Here's how the part is built. I have some questions about the finished solid (model axes, mm). Coordinates: 2 decimals unless noted, no trailing zeros. Write each loop counter-clockwise with the first axis right and the second up, starting at its lowest first coordinate (ties: lowest second). Pieces come first, ordered by that corner, then holes. Notation, with made-up numbers: (44, 50.5) -> (61, 50.5) arc R27 ccw to (61, 81.5) -> close; hole circle Ø11 at (48, 0.25). An arc over 180 degrees is marked (long way). Use a Markdown table: item, result. Add a question column.
Item 1: Imagine slicing it at B-B, the plane y = 0. Write out the boundary of the cut face in (x, z).
Item 2: Will this pin go through, and if not, where does the flat tip stop? pin 1 Ø6.5 at (y, z) = (0, 12.7) entering from -X.
Item 3: Imagine slicing it at A-A, the plane z = 352.7. Write out the boundary of the cut face in (x, y), and give its area (3 significant figures).
Item 4: If I drill on line 1 along Y through (x, z) = (0.75, 352.7); line 2 along Z through (x, y) = (-11.25, 1.5); line 3 along Z through (x, y) = (-1.25, 2.25), over which ranges is the centre line in solid material (lowest first)? Write a range as from..to.
Item 5: If we mould it in two halves opening along Y, with no side actions, what happens to faces 1 (the flat face through (0, 12.7, 180)), 2 (the flat face through (0, 0, 365.4)), 3 (the cylindrical face through (-0.18, 1.05, 356.04))? For each: pulls with the +Y half, pulls with the -Y half, needs draft (parallel to the pull), parting line crosses it, or undercut.
```python
from build123d import *

# Parameters (mm, degrees)
SKETCH1_W           = 25.4
SKETCH1_H           = 25.4
BOSS_EXTRUDE1_DEPTH = 365.4
SKETCH10_R          = 3.5
CUT_EXTRUDE6_DEPTH  = 367.501855384


with BuildPart() as part:
    # Sketch1 → Boss-Extrude1 (new body)
    with BuildSketch(Plane.XY):
        Rectangle(SKETCH1_W, SKETCH1_H)
    extrude(amount=BOSS_EXTRUDE1_DEPTH)

    # Sketch10 → Cut-Extrude6 (cut, through all)
    with BuildSketch(Plane.ZY.offset(12.7)):
        with Locations((352.7, 0)):
            Circle(SKETCH10_R)
        with Locations(Location((12.7, 0, 0), (0, 0, 180))):
            Circle(SKETCH10_R)
    extrude(amount=-CUT_EXTRUDE6_DEPTH, mode=Mode.SUBTRACT)


solid = part.part
```
Ans:
| question | item | result |
|---|---|---|
| 1 | outline | (-12.7, 0) -> (12.7, 0) -> (12.7, 9.2) -> (-12.7, 9.2) -> close; (-12.7, 16.2) -> (12.7, 16.2) -> (12.7, 349.2) -> (-12.7, 349.2) -> close; (-12.7, 356.2) -> (12.7, 356.2) -> (12.7, 365.4) -> (-12.7, 365.4) -> close |
| 2 | pin 1 | passes through |
| 3 | outline | (-12.7, -12.7) -> (12.7, -12.7) -> (12.7, -3.5) -> (-12.7, -3.5) -> close; (-12.7, 3.5) -> (12.7, 3.5) -> (12.7, 12.7) -> (-12.7, 12.7) -> close |
| 3 | area | 467 mm^2 |
| 4 | line 1 | y = -12.7..-3.5, 3.5..12.7 |
| 4 | line 2 | z = 0..9.54, 15.86..349.54, 355.86..365.4 |
| 4 | line 3 | z = 0..10.02, 15.38..350.02, 355.38..365.4 |
| 5 | face 1 | pulls with the +Y half |
| 5 | face 2 | needs draft |
| 5 | face 3 | undercut |
